```python
from build123d import *

# Parameters (mm, degrees)
SKETCH_1_W          = 210
SKETCH_1_H          = 115
EXTRUDE_6_DEPTH     = 6.75
FILLET_6_R          = 7
FILLET_7_R          = 4
SHELL_6_T           = 3
SKETCH_10_W         = 85
SKETCH_10_H         = 55.5
CUT_EXTRUDE_1_DEPTH = 125.175690155
SKETCH_11_R         = 6.5
SKETCH_11_W         = 9
SKETCH_11_H         = 9
CUT_EXTRUDE_2_DEPTH = 125.175690155
SKETCH_12_R         = 4.5
SKETCH_12_R_2       = 1.5
EXTRUDE_9_DEPTH     = 6


with BuildPart() as part:
    # Эскиз1 → Бобышка-Вытянуть6 (new body)
    with BuildSketch(Plane.XY):
        Rectangle(SKETCH_1_W, SKETCH_1_H)
    extrude(amount=EXTRUDE_6_DEPTH)

    # Скругление6
    # the kernel refuses this fillet: 7 mm, written as the material it takes off along each edge
    with BuildSketch(Plane(origin=(105, 74.988835725, 6.75), x_dir=(0, 0, -1), z_dir=(0, -1, 0)), Plane(origin=(-105, -74.988835725, 6.75), x_dir=(0, 0, -1), z_dir=(0, 1, 0))) as fillet_6_piece_1:
        with BuildLine():
            CenterArc((7, -6.99553429), FILLET_6_R, 92.046713098, 87.953286902)
            Line((0, -6.99553429), (-0.14, -6.99553429))
            Line((-0.14, -6.99553429), (-0.14, 0))
            Line((-0.14, 0), (0, 0.14))
            ThreePointArc((0, 0.14), (3.375, 0.14), (6.745, 0.139910686))
            Line((6.745, 0.139910686), (6.75, 0))
        make_face()
    extrude(amount=149.977671449, mode=Mode.SUBTRACT)

    # Скругление7
    fillet_7_edges = [part.edges().sort_by_distance(p)[0] for p in [
        (0, -57.5, 6.75),
        (0, 57.5, 6.75),
        (-102.865021234, 57.5, 4.78736042),
        (102.865021234, 57.5, 4.78736042),
        (-102.865021234, -57.5, 4.78736042),
        (102.865021234, -57.5, 4.78736042),
    ]]
    fillet(fillet_7_edges, radius=FILLET_7_R)

    # Оболочка6
    shell_6_openings = [part.faces().sort_by_distance(p)[0] for p in [
        (0, -1.3e-08, 0),
    ]]
    offset(amount=SHELL_6_T, openings=shell_6_openings, kind=Kind.INTERSECTION)

    # Эскиз10 → Вырез-Вытянуть1 (cut, through all)
    with BuildSketch(Plane.XY.offset(9.75)):
        with Locations((0, 18.25)):
            Rectangle(SKETCH_10_W, SKETCH_10_H)
    extrude(amount=-CUT_EXTRUDE_1_DEPTH, mode=Mode.SUBTRACT)

    # Эскиз11 → Вырез-Вытянуть2 (cut, through all)
    with BuildSketch(Plane.XY.offset(9.75)):
        with Locations((-44, -28)):
            Circle(SKETCH_11_R)
        with Locations((-55.5, -39.5)):
            Circle(SKETCH_11_R)
        with Locations((-55.5, -16.5)):
            Circle(SKETCH_11_R)
        with Locations((-67, -28)):
            Circle(SKETCH_11_R)
        with Locations((51.25, -18.5)):
            Circle(SKETCH_11_R)
        with Locations((62.75, -30)):
            Circle(SKETCH_11_R)
        with Locations((51.25, -41.5)):
            Circle(SKETCH_11_R)
        with Locations((39.75, -30)):
            Circle(SKETCH_11_R)
        with Locations((-62.5, 12)):
            Circle(SKETCH_11_R)
        with Locations((60.25, 17.5)):
            Rectangle(SKETCH_11_W, SKETCH_11_H)
    extrude(amount=-CUT_EXTRUDE_2_DEPTH, mode=Mode.SUBTRACT)

    # Эскиз12 → Бобышка-Вытянуть9 (add)
    # profile 1 of 4: a face of its own
    with BuildSketch(Plane(origin=(0, 0, 6.75), x_dir=(-1, 0, 0), z_dir=(0, 0, -1))):
        with Locations(Location((74, 37.5, 0), (0, 0, 180))):
            Circle(SKETCH_12_R)
        with Locations((74, 37.5)):
            Circle(SKETCH_12_R_2, mode=Mode.SUBTRACT)
    # profile 2 of 4: a face of its own
    with BuildSketch(Plane(origin=(0, 0, 6.75), x_dir=(-1, 0, 0), z_dir=(0, 0, -1))):
        with Locations(Location((-68.75, 37.5, 0), (0, 0, 180))):
            Circle(SKETCH_12_R)
        with Locations((-68.75, 37.5)):
            Circle(SKETCH_12_R_2, mode=Mode.SUBTRACT)
    # profile 3 of 4: a face of its own
    with BuildSketch(Plane(origin=(0, 0, 6.75), x_dir=(-1, 0, 0), z_dir=(0, 0, -1))):
        with Locations(Location((74, -44.75, 0), (0, 0, 180))):
            Circle(SKETCH_12_R)
        with Locations((74, -44.75)):
            Circle(SKETCH_12_R_2, mode=Mode.SUBTRACT)
    # profile 4 of 4: a face of its own
    with BuildSketch(Plane(origin=(0, 0, 6.75), x_dir=(-1, 0, 0), z_dir=(0, 0, -1))):
        with Locations(Location((-68.75, -44.75, 0), (0, 0, 180))):
            Circle(SKETCH_12_R)
        with Locations((-68.75, -44.75)):
            Circle(SKETCH_12_R_2, mode=Mode.SUBTRACT)
    extrude(amount=EXTRUDE_9_DEPTH)


solid = part.part
```
Input: part model. Units: mm. Frame: model coordinates. A direction names the side the tool comes from. Coordinates: 2 decimals unless noted, no trailing zeros. Write each loop counter-clockwise with the first axis right and the second up, starting at its lowest first coordinate (ties: lowest second). Pieces come first, ordered by that corner, then holes. Notation, with made-up numbers: M 45,30.25 L 69,30.25 A22 cw 69,39.25 Z; hole C 17.25,-40 d5. An arc over 180 degrees is marked long. Use one line per item in the form item = value.
Q1. Draft query along X for faces 3 (the face through (-105.064, -0.749, 6.833)), 4 (the face through (68, 36, 0.75)), 5 (the face through (105.064, 0.749, 6.833)), 6 (the face through (-1, 59, 0)). Return one class per face: released by +X, released by -X, zero draft, split by the parting line, or undercut.
Answer below:
face_3 = released by -X
face_4 = undercut
face_5 = released by +X
face_6 = zero draft
Q2. First-contact query: pin 1 (4.5 mm diameter, centred on x = 70, y = -45, fed in from -Z); pin 2 (1.5 mm diameter, centred on y = 15.5, z = 8, fed in from -X); pin 3 (1.5 mm diameter, centred on y = 16.5, z = 8.5, fed in from +X). Flat tips, straight axial feed; report the tip coordinate or a pass-through.
Answer below:
pin_1 = 0.75
pin_2 = -104.62
pin_3 = 104
Q3. Section C-C (y = -28). Return loops of the section in (x, z), plus the area to 3 significant figures.
Answer below:
outline = M -108,0 L -105,0 A7 cw -98,6.75 L -73.5,6.75 L -73.5,9.75 L -98,9.75 A10 ccw Z; M -60.5,6.75 L -50.5,6.75 L -50.5,9.75 L -60.5,9.75 Z; M -37.5,6.75 L 33.57,6.75 L 33.57,9.75 L -37.5,9.75 Z; M 45.93,6.75 L 56.57,6.75 L 56.57,9.75 L 45.93,9.75 Z; M 68.93,6.75 L 98,6.75 A7 cw 105,0 L 108,0 A10 ccw 98,9.75 L 68.93,9.75 Z
area = 514 mm²
Q4. Section D-D (x = 90.5). Return loops of the section in (y, z).
Answer below:
outline = M -60.5,0 L -57.5,0 L -57.5,2.75 A4 cw -53.5,6.75 L 53.5,6.75 A4 cw 57.5,2.75 L 57.5,0 L 60.5,0 L 60.5,2.75 A7 ccw 53.5,9.75 L -53.5,9.75 A7 ccw -60.5,2.75 Z
Q5. Section B-B (y = 31). Return loops of the section in (x, z).
Answer below:
outline = M -108,0 L -105,0 A7 cw -98,6.75 L -42.5,6.75 L -42.5,9.75 L -98,9.75 A10 ccw Z; M 42.5,6.75 L 98,6.75 A7 cw 105,0 L 108,0 A10 ccw 98,9.75 L 42.5,9.75 Z
Q6. Material intervals for probe 1 along Y at (x, z) = (77, 1.75); probe 2 along Y at (x, z) = (-74, 4.45); probe 3 along Y at (x, z) = (69, 5.75), sorted ascending. Write a range as from..to.
Answer below:
probe_1 = -60.5..-57.5, 57.5..60.5
probe_2 = -60.29..-57.12, -49.25..-46.25, -43.25..-40.25, 33..36, 39..42, 57.12..60.29
probe_3 = -59.82..-56.15, -49.24..-46.23, -43.27..-40.26, 33.01..36.02, 38.98..41.99, 56.15..59.82
Q7. Section A-A (x = 8). Return loops of the section in (y, z).
Answer below:
outline = M -60.5,0 L -57.5,0 L -57.5,2.75 A4 cw -53.5,6.75 L -9.5,6.75 L -9.5,9.75 L -53.5,9.75 A7 ccw -60.5,2.75 Z; M 46,6.75 L 53.5,6.75 A4 cw 57.5,2.75 L 57.5,0 L 60.5,0 L 60.5,2.75 A7 ccw 53.5,9.75 L 46,9.75 Z
Q8. Set-up query: faces 1 (the face through (-75, 36, 0.75)), 2 (the face through (1.37, -58.5, 7.65)). Return all of +Z, -Z, +X, -X, +Y, -Y with unobstructed straight access to the full face (end or side cutting, diameter ignored); none if empty.
Answer below:
face_1 = -Z
face_2 = +Z, +X, -X, -Y
